```python
from build123d import *

# Parameters (mm, degrees)
EXTRUDE_THIN1_START          = -6.35
EXTRUDE_THIN1_DEPTH          = 12.7
SKETCH4_R                    = 2.3495
EXTRUDE3_DEPTH               = 51.526212207
SKETCH7_R                    = 3.5433
CUT_EXTRUDE1_DEPTH           = 54.020940995
CUT_EXTRUDE1_DRAFT           = -49
CUT_EXTRUDE1_PROFILE_2_DEPTH = 54.020940995
CUT_EXTRUDE1_PROFILE_2_DRAFT = -49
CIRPATTERN1_COUNT            = 2
CIRPATTERN1_COPY_1_SKETCH_R  = 3.5433
CIRPATTERN1_COPY_1_DEPTH     = 54.020940995
CIRPATTERN1_COPY_1_DRAFT     = -49
CIRPATTERN1_COPY_2_SKETCH_R  = 3.5433
CIRPATTERN1_COPY_2_DEPTH     = 54.020940995
CIRPATTERN1_COPY_2_DRAFT     = -49
CIRPATTERN1_COPY_3_SKETCH_R  = 3.5433
CIRPATTERN1_COPY_3_DEPTH     = 54.020940995
CIRPATTERN1_COPY_3_DRAFT     = -49


# Read off the part's stored shape, not the designer's step: Extrude-Thin1
with BuildPart() as part:
    # Extrude-Thin1 outline → Extrude-Thin1 (new body)
    with BuildSketch(Plane(origin=(0, 0, 0), x_dir=(1, 0, 0), z_dir=(0, 1, 0)).offset(EXTRUDE_THIN1_START)):
        with BuildLine():
            Line((2.667, -1.778), (38.1, -1.778))
            Line((38.1, -1.778), (38.1, 0))
            Line((38.1, 0), (2.667, 0))
            ThreePointArc((2.667, 0), (0.781146215, -0.781146215), (0, -2.667))
            Line((0, -2.667), (0, -38.1))
            Line((0, -38.1), (1.778, -38.1))
            Line((1.778, -38.1), (1.778, -2.667))
            ThreePointArc((1.778, -2.667), (2.038382072, -2.038382072), (2.667, -1.778))
        make_face()
    extrude(amount=EXTRUDE_THIN1_DEPTH)

    # Sketch4 → Extrude3 (cut, through all)
    with BuildSketch(Plane(origin=(3.556, 0, 1.778), x_dir=(1, 0, 0), z_dir=(0, 0, 1))):
        with Locations((27.432, 0)):
            Circle(SKETCH4_R)
        with Locations((8.89, 0)):
            Circle(SKETCH4_R)
    extrude3 = extrude(amount=-EXTRUDE3_DEPTH, mode=Mode.SUBTRACT)


with BuildPart() as cut_extrude1_tool:
    # Sketch7 → Cut-Extrude1 (with draft: the straight prism first)
    with BuildSketch(Plane.XY.offset(1.778)):
        with Locations((30.988, 0)):
            Circle(SKETCH7_R)
    extrude(amount=-CUT_EXTRUDE1_DEPTH)
    # Cut-Extrude1: the draft: its side faces are tilted about the plane it starts from
    cut_extrude1_sides = [cut_extrude1_tool.faces().sort_by_distance(p)[0] for p in [
        (27.4447, 0, -25.232470498),
    ]]
    draft(cut_extrude1_sides, Plane.XY.offset(1.778), CUT_EXTRUDE1_DRAFT)


with BuildPart() as part_1:
    add(part.part)

    # Cut-Extrude1: cut by cut_extrude1_tool
    add(cut_extrude1_tool.part, mode=Mode.SUBTRACT)


with BuildPart() as cut_extrude1_profile_2_tool:
    # Sketch7 → Cut-Extrude1 profile 2 (with draft: the straight prism first)
    with BuildSketch(Plane.XY.offset(1.778)):
        with Locations((12.446, 0)):
            Circle(SKETCH7_R)
    extrude(amount=-CUT_EXTRUDE1_PROFILE_2_DEPTH)
    # Cut-Extrude1 profile 2: the draft: its side faces are tilted about the plane it starts from
    cut_extrude1_profile_2_sides = [cut_extrude1_profile_2_tool.faces().sort_by_distance(p)[0] for p in [
        (8.9027, 0, -25.232470498),
    ]]
    draft(cut_extrude1_profile_2_sides, Plane.XY.offset(1.778), CUT_EXTRUDE1_PROFILE_2_DRAFT)


with BuildPart() as part_2:
    add(part_1.part)

    # Cut-Extrude1 profile 2: cut by cut_extrude1_profile_2_tool
    add(cut_extrude1_profile_2_tool.part, mode=Mode.SUBTRACT)

    # CirPattern1: Extrude3 ×2 about axis
    cirpattern1_axis = Axis((0, 0, 0), (0.7071067811865464, 0, 0.7071067811865487))
    for i in range(1, CIRPATTERN1_COUNT):
        add(extrude3.rotate(cirpattern1_axis, i * 360 / CIRPATTERN1_COUNT), mode=Mode.SUBTRACT)


with BuildPart() as cirpattern1_copy_1_tool:
    # CirPattern1 copy 1 sketch → CirPattern1 copy 1 (with draft: the straight prism first)
    with BuildSketch(Plane(origin=(1.778, 0, 0), x_dir=(0, 0, 1), z_dir=(1, 0, 0))):
        with Locations((30.988, 0)):
            Circle(CIRPATTERN1_COPY_1_SKETCH_R)
    extrude(amount=-CIRPATTERN1_COPY_1_DEPTH)
    # CirPattern1 copy 1: the draft: its side faces are tilted about the plane it starts from
    cirpattern1_copy_1_sides = [cirpattern1_copy_1_tool.faces().sort_by_distance(p)[0] for p in [
        (-25.232470498, 0, 27.4447),
    ]]
    draft(cirpattern1_copy_1_sides, Plane(origin=(1.778, 0, 0), x_dir=(0, 0, 1), z_dir=(1, 0, 0)), CIRPATTERN1_COPY_1_DRAFT)


with BuildPart() as part_3:
    add(part_2.part)

    # CirPattern1 copy 1: cut by cirpattern1_copy_1_tool
    add(cirpattern1_copy_1_tool.part, mode=Mode.SUBTRACT)


with BuildPart() as cirpattern1_copy_2_tool:
    # CirPattern1 copy 2 sketch → CirPattern1 copy 2 (with draft: the straight prism first)
    with BuildSketch(Plane(origin=(1.778, 0, 0), x_dir=(0, 0, 1), z_dir=(1, 0, 0))):
        with Locations((12.446, 0)):
            Circle(CIRPATTERN1_COPY_2_SKETCH_R)
    extrude(amount=-CIRPATTERN1_COPY_2_DEPTH)
    # CirPattern1 copy 2: the draft: its side faces are tilted about the plane it starts from
    cirpattern1_copy_2_sides = [cirpattern1_copy_2_tool.faces().sort_by_distance(p)[0] for p in [
        (-25.232470498, 0, 8.9027),
    ]]
    draft(cirpattern1_copy_2_sides, Plane(origin=(1.778, 0, 0), x_dir=(0, 0, 1), z_dir=(1, 0, 0)), CIRPATTERN1_COPY_2_DRAFT)


with BuildPart() as part_4:
    add(part_3.part)

    # CirPattern1 copy 2: cut by cirpattern1_copy_2_tool
    add(cirpattern1_copy_2_tool.part, mode=Mode.SUBTRACT)


with BuildPart() as cirpattern1_copy_3_tool:
    # CirPattern1 copy 3 sketch → CirPattern1 copy 3 (with draft: the straight prism first)
    with BuildSketch(Plane(origin=(1.778, 0, 0), x_dir=(0, 0, 1), z_dir=(1, 0, 0))):
        with Locations((12.446, 0)):
            Circle(CIRPATTERN1_COPY_3_SKETCH_R)
    extrude(amount=-CIRPATTERN1_COPY_3_DEPTH)
    # CirPattern1 copy 3: the draft: its side faces are tilted about the plane it starts from
    cirpattern1_copy_3_sides = [cirpattern1_copy_3_tool.faces().sort_by_distance(p)[0] for p in [
        (-25.232470498, 0, 8.9027),
    ]]
    draft(cirpattern1_copy_3_sides, Plane(origin=(1.778, 0, 0), x_dir=(0, 0, 1), z_dir=(1, 0, 0)), CIRPATTERN1_COPY_3_DRAFT)


with BuildPart() as part_5:
    add(part_4.part)

    # CirPattern1 copy 3: cut by cirpattern1_copy_3_tool
    add(cirpattern1_copy_3_tool.part, mode=Mode.SUBTRACT)


solid = part_5.part
```
Check sheet for the modelled part. Datum: model origin and axes. Units: mm. A direction names the side the tool comes from. Round coordinates to 2 decimals unless told otherwise and drop trailing zeros. Order: outer loops, then holes, each group sorted by start corner. A loop starts at its lowest first (then second) coordinate and runs counter-clockwise, first axis right, second up. Notation, with made-up numbers: (6.5, 40) -> (13.5, 40) arc R24 ccw to (13.5, 58) -> close; hole circle Ø5 at (-10, 15.5). An arc over 180 degrees is marked (long way). Use CSV: the item, a comma, the result in double quotes.
(1) Material ranges on line 1 along X through (y, z) = (1.5, 7); line 2 along X through (y, z) = (1.75, 10), recorded low to high. Write a range as from..to.
Worked out:
line 1,"0..1.78"
line 2,"0..1.31"
(2) Cross-section at C-C (z = 20). Record the boundary of the cut face in (x, y), and give its area (3 significant figures).
Worked out:
outline,"(0, -6.35) -> (1.78, -6.35) -> (1.78, 6.35) -> (0, 6.35) -> close"
area,"22.6 mm²"
(3) Tool access check on faces 1 (the face through (0.8, -0.09, 0.76)), 2 (the face through (1.778, 0, 21)). Record the directions out of +Z, -Z, +X, -X, +Y, -Y that give a thin tool (end or side, any length) a straight path to the whole face; none if there is none.
Worked out:
face 1,"-Z, -X, +Y, -Y"
face 2,"+Z, +X, +Y, -Y"
(4) Cross-section at D-D (x = 19). Record the boundary of the cut face in (y, z), and give its area (3 significant figures).
Worked out:
outline,"(-6.35, 0) -> (6.35, 0) -> (6.35, 1.78) -> (-6.35, 1.78) -> close"
area,"22.6 mm²"
(5) Depth check by flat-ended pin: pin 1 (7.5 mm diameter, centred on y = 0, z = 30.988, fed in from -X); pin 2 (6 mm diameter, centred on y = 0, z = 12.446, fed in from +X); pin 3 (3 mm diameter, centred on y = 3, z = 6.5, fed in from +X); pin 4 (5.5 mm diameter, centred on x = 30.988, y = 0, fed in from +Z). Enter the tip coordinate at first touch or a pass-through.
Worked out:
pin 1,"x = 0"
pin 2,"x = 1.31"
pin 3,"x = 1.78"
pin 4,"z = 1.09"
(6) Cross-section at B-B (y = -4.75). Record the boundary of the cut face in (x, z), and give its area (3 significant figures).
Worked out:
outline,"(0, 2.67) arc R2.67 ccw to (2.67, 0) -> (38.1, 0) -> (38.1, 1.78) -> (2.67, 1.78) arc R0.89 cw to (1.78, 2.67) -> (1.78, 38.1) -> (0, 38.1) -> close"
area,"131 mm²"
(7) Cross-section at A-A (y = 0). Count the separate pieces of the cut face and the enclosed holes in it, and give its area (3 significant figures).
Worked out:
separate pieces,"5"
enclosed holes,"0"
area,"92.6 mm²"
(8) Draft check along Z on faces 3 (the face through (0.375, -0.706, 33.229)), 4 (the face through (1, 0, 38.1)), 5 (the face through (0.4, -0.1, 10.1)), 6 (the face through (33.229, 0.706, 0.375)). Enter one of: pulls with the +Z half, pulls with the -Z half, needs draft (parallel to the pull), parting line crosses it, or undercut.
Worked out:
face 3,"undercut"
face 4,"pulls with the +Z half"
face 5,"undercut"
face 6,"needs draft"
